Read the model definition and answer for the solid it produces. Units are mm, in the model's axes. Coordinates: 2 decimals unless noted, no trailing zeros. Order: outer loops, then holes, each group sorted by start corner. A loop starts at its lowest first (then second) coordinate and runs counter-clockwise, first axis right, second up. Notation, with made-up numbers: (70.25, -20.5) -> (117.25, -20.5) arc R26 ccw to (117.25, 1.5) -> close; hole circle Ø10 at (-27, 63.5). An arc over 180 degrees is marked (long way). Use CSV: the item, a comma, the result in double quotes.
```python
from build123d import *

# Parameters (mm, degrees)
F0_W     = 50
F0_H     = 280
F1_DEPTH = 3
F2_W     = 3
F2_H     = 20
F3_DEPTH = 25
F4_W     = 7.5
F4_H     = 3
F5_DEPTH = 25
F7_DEPTH = 3


with BuildPart() as f1:
    # F0 (on Top) → F1 (new body)
    with BuildSketch(Plane.XY):
        Rectangle(F0_W, F0_H)
    extrude(amount=F1_DEPTH)

    # F2 (on face) → F3 (cut)
    with BuildSketch(Plane.XY.offset(3)):
        with Locations((3, 120)):
            Rectangle(F2_W, F2_H)
        with Locations((3, 80)):
            Rectangle(F2_W, F2_H)
        with Locations((3, 40)):
            Rectangle(F2_W, F2_H)
        with Locations((3, 0)):
            Rectangle(F2_W, F2_H)
        with Locations((3, -40)):
            Rectangle(F2_W, F2_H)
        with Locations((3, -80)):
            Rectangle(F2_W, F2_H)
        with Locations((3, -120)):
            Rectangle(F2_W, F2_H)
        with Locations((-3, 120)):
            Rectangle(F2_W, F2_H)
        with Locations((-3, 80)):
            Rectangle(F2_W, F2_H)
        with Locations((-3, 40)):
            Rectangle(F2_W, F2_H)
        with Locations((-3, 0)):
            Rectangle(F2_W, F2_H)
        with Locations((-3, -40)):
            Rectangle(F2_W, F2_H)
        with Locations((-3, -80)):
            Rectangle(F2_W, F2_H)
        with Locations((-3, -120)):
            Rectangle(F2_W, F2_H)
    extrude(amount=-F3_DEPTH, mode=Mode.SUBTRACT)

    # F4 (on face) → F5 (cut)
    with BuildSketch(Plane.XY.offset(3)):
        with Locations((15.75, 120)):
            Rectangle(F4_W, F4_H)
        with Locations((15.75, 80)):
            Rectangle(F4_W, F4_H)
        with Locations((15.75, 40)):
            Rectangle(F4_W, F4_H)
        with Locations((15.75, 0)):
            Rectangle(F4_W, F4_H)
        with Locations((15.75, -40)):
            Rectangle(F4_W, F4_H)
        with Locations((15.75, -80)):
            Rectangle(F4_W, F4_H)
        with Locations((15.75, -120)):
            Rectangle(F4_W, F4_H)
        with Locations((-15.75, 120)):
            Rectangle(F4_W, F4_H)
        with Locations((-15.75, -80)):
            Rectangle(F4_W, F4_H)
        with Locations((-15.75, 40)):
            Rectangle(F4_W, F4_H)
        with Locations((-15.75, 80)):
            Rectangle(F4_W, F4_H)
        with Locations((-15.75, -40)):
            Rectangle(F4_W, F4_H)
        with Locations((-15.75, -120)):
            Rectangle(F4_W, F4_H)
        with Locations((-15.75, 0)):
            Rectangle(F4_W, F4_H)
    extrude(amount=-F5_DEPTH, mode=Mode.SUBTRACT)

    # F6 (on face) → F7 (join)
    with BuildSketch(Plane.XY.offset(3)):
        with BuildLine():
            ThreePointArc((25, 153.005103), (0, 142.5), (-25, 153.005103))
            Line((-25, 153.005103), (-25, 140))
            Line((-25, 140), (25, 140))
            Line((25, 140), (25, 153.005103))
        make_face()
        with BuildLine():
            Line((25, -140), (-25, -140))
            Line((-25, -140), (-25, -153.005103))
            ThreePointArc((-25, -153.005103), (0, -142.5), (25, -153.005103))
            Line((25, -153.005103), (25, -140))
        make_face()
    extrude(amount=-F7_DEPTH)


solid = f1.part
```
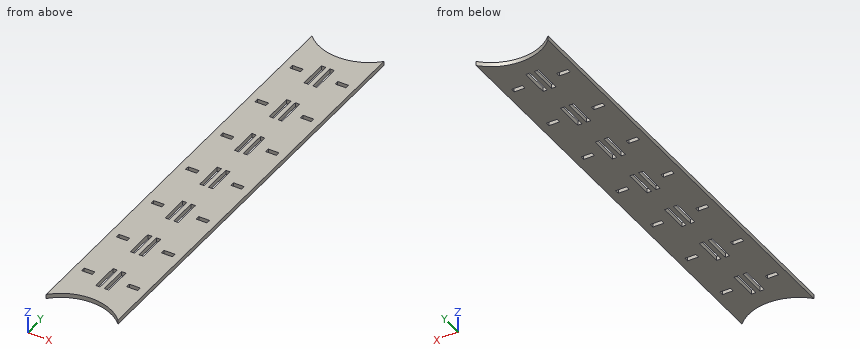
Item 1: Each of these flat-tipped pins is pushed along its axis until it touches: P1, Ø1.5, axis at x = 3.5, z = 1, coming from the +Y side; P2, Ø0.9, axis at x = -2.5, z = 1, coming from the +Y side; P3, Ø0.9, axis at x = 14, z = 1.5, coming from the -Y side. Where does it stop, or does it pass through?
Return value:
P1,"stops at y = 142.76"
P2,"stops at y = 142.62"
P3,"stops at y = -145.62"
Item 2: Find section A-A, the plane y = -4.5. Give the vertices of the cut face in (x, z), then the cut area to 3 significant figures.
Return value:
outline,"(-25, 0) -> (-4.5, 0) -> (-4.5, 3) -> (-25, 3) -> close; (-1.5, 0) -> (1.5, 0) -> (1.5, 3) -> (-1.5, 3) -> close; (4.5, 0) -> (25, 0) -> (25, 3) -> (4.5, 3) -> close"
area,"132 mm^2"
Item 3: Find section B-B, the plane x = 14.5. Give the number of separate pieces and of enclosed holes in the cut face, then the cut area to 3 significant figures.
Return value:
separate pieces,"8"
enclosed holes,"0"
area,"811 mm^2"
Item 4: Straight lines are drawn through the part: line 1 along X through (y, z) = (9.5, 0.95); line 2 along X through (y, z) = (-79, 1.6); line 3 along Y through (x, z) = (-9, 0.55). For each, find the intervals that lie inside material, in ascending order.
Return value:
line 1,"x = -25 to -4.5, -1.5 to 1.5, 4.5 to 25"
line 2,"x = -25 to -19.5, -12 to -4.5, -1.5 to 1.5, 4.5 to 12, 19.5 to 25"
line 3,"y = -143.68 to 143.68"
